```python
from build123d import *

# Parameters (mm, degrees)
F0_W     = 56.388
F0_H     = 56.388
F1_DEPTH = 111.99876
F2_R     = 2.49936
F3_DEPTH = 111.99976
F4_R     = 19.05
F5_DEPTH = 1.59766
F6_R     = 3.97383
F7_DEPTH = 25.4
F9_DEPTH = 103.886
F10_R    = 2.54


with BuildPart() as f1:
    # F0 (on Top) → F1 (new body)
    with BuildSketch(Plane.XY):
        Rectangle(F0_W, F0_H)
    extrude(amount=F1_DEPTH)

    # F2 (on face) → F3 (cut, through all)
    with BuildSketch(Plane.XY.offset(111.99876)):
        with Locations((-23.56993, 23.273565)):
            Circle(F2_R)
        with Locations((23.56993, 23.273565)):
            Circle(F2_R)
        with Locations((23.56993, -23.273565)):
            Circle(F2_R)
        with Locations((-23.56993, -23.273565)):
            Circle(F2_R)
    extrude(amount=-F3_DEPTH, mode=Mode.SUBTRACT)

    # F4 (on face) → F5 (join)
    with BuildSketch(Plane.XY.offset(111.99876)):
        Circle(F4_R)
    extrude(amount=F5_DEPTH)

    # F6 (on face) → F7 (join)
    with BuildSketch(Plane.XY.offset(113.59642)):
        Circle(F6_R)
    extrude(amount=F7_DEPTH)

    # F8 (on face) → F9 (cut)
    with BuildSketch(Plane(origin=(0, 0, 0), x_dir=(1, 0, 0), z_dir=(0, 0, -1))):
        with BuildLine():
            ThreePointArc((-23.594014, 18.158077), (-19.910458, 19.713716), (-18.457055, 23.438796))
            Line((-18.457055, 23.438796), (-18.610727, 28.194))
            Line((-18.610727, 28.194), (-28.194, 28.194))
            Line((-28.194, 28.194), (-28.194, 18.158077))
            Line((-28.194, 18.158077), (-23.594014, 18.158077))
        make_face()
        with BuildLine():
            Line((-18.704263, -28.194), (-18.704263, -23.265395))
            ThreePointArc((-18.704263, -23.265395), (-20.132269, -19.830127), (-23.56993, -18.407891))
            Line((-23.56993, -18.407891), (-28.194, -18.407891))
            Line((-28.194, -18.407891), (-28.194, -28.194))
            Line((-28.194, -28.194), (-18.704263, -28.194))
        make_face()
        with BuildLine():
            ThreePointArc((23.56993, -18.27852), (20.009329, -19.770338), (18.575544, -23.3547))
            Line((18.575544, -23.3547), (18.575544, -28.194))
            Line((18.575544, -28.194), (28.194, -28.194))
            Line((28.194, -28.194), (28.194, -18.27852))
            Line((28.194, -18.27852), (23.56993, -18.27852))
        make_face()
        with BuildLine():
            Line((18.663428, 28.194), (18.663428, 23.151265))
            ThreePointArc((18.663428, 23.151265), (20.142944, 19.760093), (23.56993, 18.365539))
            Line((23.56993, 18.365539), (28.194, 18.365539))
            Line((28.194, 18.365539), (28.194, 28.194))
            Line((28.194, 28.194), (18.663428, 28.194))
        make_face()
    extrude(amount=-F9_DEPTH, mode=Mode.SUBTRACT)

    # F10
    f10_edges = [f1.edges().sort_by_distance(p)[0] for p in [
        (-28.194, 0.124907, 0),
        (0.026351, -28.194, 0),
        (28.194, -0.04351, 0),
        (-0.06436, 28.194, 0),
    ]]
    fillet(f10_edges, radius=F10_R)


solid = f1.part
```
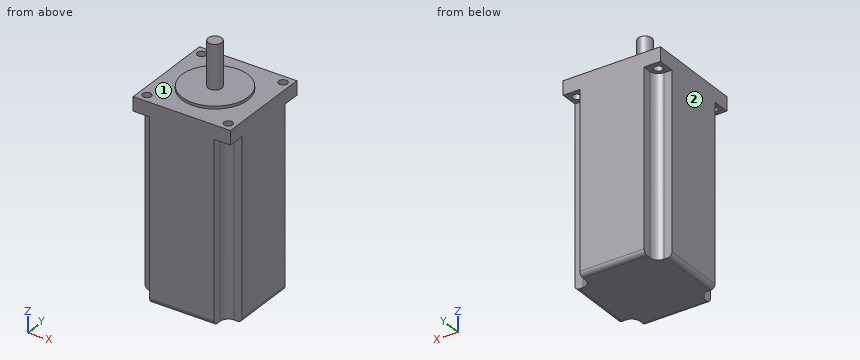
Input: part model. Units: mm. Frame: model coordinates. Face numbers are marked on the shaded views. A direction names the side the tool comes from. Give positions to 0.01 mm unless a question says otherwise; leave off trailing zeros. Write each loop counter-clockwise with the first axis right and the second up, starting at its lowest first coordinate (ties: lowest second). Pieces come first, ordered by that corner, then holes. Notation, with made-up numbers: (9, -29) - (52, -29) arc R20 ccw to (52, 1) - close; hole circle Ø3 at (66, 46.5). An arc over 180 degrees is marked (long way). Write item = value, one per line. Start each with the question number.
1) Cut plane B-B (y = 0). Return loops of the section in (x, z).
2) Cut plane D-D (y = 8.5). Return loops of the section in (x, z), and give its area (3 significant figures).
3) Cut plane A-A (z = 64.5). Return loops of the section in (x, y), and give its area (3 significant figures).
4) Pin query (flat end, axial travel): pin 1 (1.4 mm diameter, centred on x = -25, z = 53, fed in from -Y); pin 2 (5.5 mm diameter, centred on x = 23.57, y = 23.27, fed in from -Z); pin 3 (1.5 mm diameter, centred on y = 26.5, z = 46, fed in from +X); pin 4 (8 mm diameter, centred on x = -8.5, y = 16.5, fed in from -Z). Return the tip coordinate at first contact, or that it passes through.
5) Reachability of the marked faces 1 and 2 from +Z, -Z, +X, -X, +Y, -Y: full face, straight path, thin tool, end or side. Return the list, or none.
6) Cut plane C-C (x = -15.5). Return loops of the section in (y, z).
7) Material intervals for L1, parallel to Z at x = -18.5, y = 14; L2, parallel to X at y = 24, z = 78.5; L3, parallel to Z at x = 1, y = 4, sorted ascending. Write a range as [from, to].
Answers follow:
q1.outline = (-28.19, 2.54) arc R2.54 ccw to (-25.65, 0) - (25.65, 0) arc R2.54 ccw to (28.19, 2.54) - (28.19, 112) - (19.05, 112) - (19.05, 113.6) - (3.97, 113.6) - (3.97, 139) - (-3.97, 139) - (-3.97, 113.6) - (-19.05, 113.6) - (-19.05, 112) - (-28.19, 112) - close
q2.outline = (-28.19, 2.54) arc R2.54 ccw to (-25.65, 0) - (25.65, 0) arc R2.54 ccw to (28.19, 2.54) - (28.19, 112) - (17.05, 112) - (17.05, 113.6) - (-17.05, 113.6) - (-17.05, 112) - (-28.19, 112) - close
q2.area = 6,370 mm^2
q3.outline = (-28.19, -18.16) - (-23.59, -18.16) arc R5.14 cw to (-18.46, -23.44) - (-18.61, -28.19) - (18.66, -28.19) - (18.66, -23.15) arc R4.91 cw to (23.57, -18.37) - (28.19, -18.37) - (28.19, 18.28) - (23.57, 18.28) arc R5 cw to (18.58, 23.35) - (18.58, 28.19) - (-18.7, 28.19) - (-18.7, 23.27) arc R4.87 cw to (-23.57, 18.41) - (-28.19, 18.41) - close
q3.area = 2,820 mm^2
q4.pin_1 = -18.16
q4.pin_2 = 103.89
q4.pin_3 = 18.58
q4.pin_4 = 0
q5.face_1 = +Z
q5.face_2 = +Z, -Z, -X, +Y, -Y
q6.outline = (-28.19, 2.54) arc R2.54 ccw to (-25.65, 0) - (25.65, 0) arc R2.54 ccw to (28.19, 2.54) - (28.19, 112) - (11.07, 112) - (11.07, 113.6) - (-11.07, 113.6) - (-11.07, 112) - (-28.19, 112) - close
q7.L1 = [0, 112]
q7.L2 = [-18.7, 18.58]
q7.L3 = [0, 113.6]
